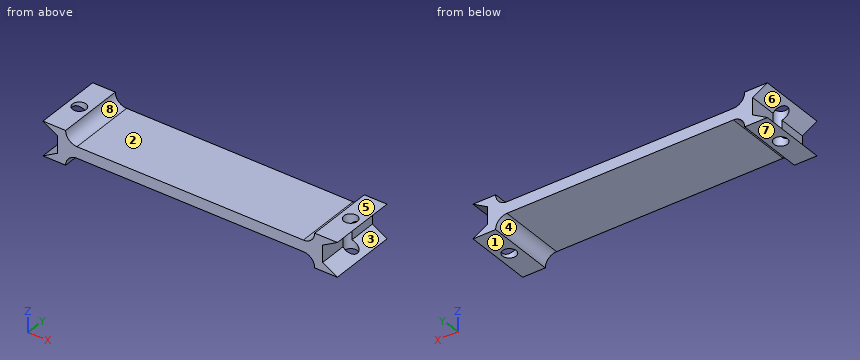
```python
from build123d import *

# Parameters (mm, degrees)
F1_DEPTH = 30
F2_R     = 3
F3_DEPTH = 15
F4_DEPTH = 50


with BuildPart() as f1:
    # F0 (on Front) → F1 (new body)
    with BuildSketch(Plane.XZ):
        with BuildLine():
            ThreePointArc((-15, -2.5), (-11.4644660941, -3.9644660941), (-10, -7.5))
            Line((-10, -7.5), (0, -7.5))
            Line((0, -7.5), (-6.4951905284, -3.75))
            Line((-6.4951905284, -3.75), (-6.4951905284, 3.75))
            Line((-6.4951905284, 3.75), (0, 7.5))
            Line((0, 7.5), (-10, 7.5))
            ThreePointArc((-10, 7.5), (-11.4644660941, 3.9644660941), (-15, 2.5))
            Line((-15, 2.5), (-15, -2.5))
        make_face()
    extrude(amount=F1_DEPTH)

    # F2 (on face) → F3 (cut, through all)
    with BuildSketch(Plane.XY.offset(7.5)):
        with Locations((-5.096135661, -15)):
            Circle(F2_R)
    extrude(amount=-F3_DEPTH, mode=Mode.SUBTRACT)

    # F4 (add): a face of the model
    f4_faces = [f1.faces().sort_by_distance(p)[0] for p in [
        (-15, -15, 0),
    ]]
    extrude(f4_faces, amount=F4_DEPTH)

    # F5: F1 across face


with BuildPart() as f1_1:
    add(f1.part)
    add(f1.part.mirror(Plane(origin=(-65, -15, 0), x_dir=(0, -1, 0), z_dir=(-1, 0, 0))))


solid = f1_1.part
```
Can you work these out from the model? Positions are in its coordinate system, mm. Face numbers are marked on the shaded views. A direction names the side the tool comes from. Coordinates: 2 decimals unless noted, no trailing zeros. Loops run counter-clockwise (first coordinate to the right, second up) from the corner with the lowest first, then second, coordinate; pieces in that order, holes last.
1) I need wall thicknesses on probe 1 along X at (y, z) = (-24, -0.5); probe 2 along Z at (x, y) = (-26.5, -6.5); probe 3 along X at (y, z) = (-5, -3). Which ranges of each line are inside material? Lowest first, please.
2) Imagine slicing it at C-C on x = -105. List the corners of the cut face in (y, z) for me.
3) For pin 1 (8 mm diameter, centred on y = -7, z = -0.5, fed in from +X); pin 2 (2 mm diameter, centred on y = -22.5, z = 0, fed in from -X); pin 3 (5 mm diameter, centred on x = -53, y = -16, fed in from +Z), each with a flat end and sliding along its axis, tell me the tip position at first contact or that it passes through.
4) Imagine slicing it at A-A on y = -6. List the corners of the cut face in (x, z) for me, plus the area to 3 significant figures.
5) Thinking about a two-plate mould opening in X: for the marked faces 1, 2 and 3, which applies, pulls with the +X half, pulls with the -X half, needs draft (parallel to the pull), parting line crosses it, or undercut?
6) Which directions (+Z, -Z, +X, -X, +Y, -Y) give clear straight access to the entire face, cutting with the end or side of a thin tool? Please do the marked faces 4, 5, 6, 7 and 8.
7) Imagine slicing it at B-B on y = -15. List the corners of the cut face in (x, z) for me.
Completed:
1. probe 1: x = -123.5 to -6.5
1. probe 2: z = -2.5 to 2.5
1. probe 3: x = -123.5 to -117.18, -12.82 to -6.5
2. outline: (-30, -2.5) - (0, -2.5) - (0, 2.5) - (-30, 2.5) - close
3. pin 1: stops at x = -5.2
3. pin 2: stops at x = -123.5
3. pin 3: stops at z = 2.5
4. outline: (-130, -7.5) - (-120, -7.5) arc R5 cw to (-115, -2.5) - (-15, -2.5) arc R5 cw to (-10, -7.5) - (0, -7.5) - (-6.5, -3.75) - (-6.5, 3.75) - (0, 7.5) - (-10, 7.5) arc R5 cw to (-15, 2.5) - (-115, 2.5) arc R5 cw to (-120, 7.5) - (-130, 7.5) - (-123.5, 3.75) - (-123.5, -3.75) - close
4. area: 725 mm2
5. face 1: needs draft
5. face 2: undercut
5. face 3: pulls with the +X half
6. face 4: -Z, +Y, -Y
6. face 5: +Z, +X, -X, +Y, -Y
6. face 6: -X, +Y, -Y
6. face 7: -Z, +X, -X, +Y, -Y
6. face 8: +Z, +Y, -Y
7. outline: (-130, -7.5) - (-127.9, -7.5) - (-127.9, -6.29) - close; (-130, 7.5) - (-127.9, 6.29) - (-127.9, 7.5) - close; (-121.9, -7.5) - (-120, -7.5) arc R5 cw to (-115, -2.5) - (-15, -2.5) arc R5 cw to (-10, -7.5) - (-8.1, -7.5) - (-8.1, 7.5) - (-10, 7.5) arc R5 cw to (-15, 2.5) - (-115, 2.5) arc R5 cw to (-120, 7.5) - (-121.9, 7.5) - close; (-2.1, -7.5) - (0, -7.5) - (-2.1, -6.29) - close; (-2.1, 6.29) - (0, 7.5) - (-2.1, 7.5) - close
